Design review of the part shown in the three views and the two pictorial views. Dimensions are in mm from the part's minimum x, y and z. A direction names the side the tool comes from. Coordinates: 2 decimals unless noted, no trailing zeros. Loops run counter-clockwise (first coordinate to the right, second up) from the corner with the lowest first, then second, coordinate; pieces in that order, holes last. Notation, with made-up numbers: (61, -27.75) -> (83, -27.75) arc R28 ccw to (83, 10.25) -> close; hole circle Ø6 at (79, 53). An arc over 180 degrees is marked (long way). One line per item, written item: value.
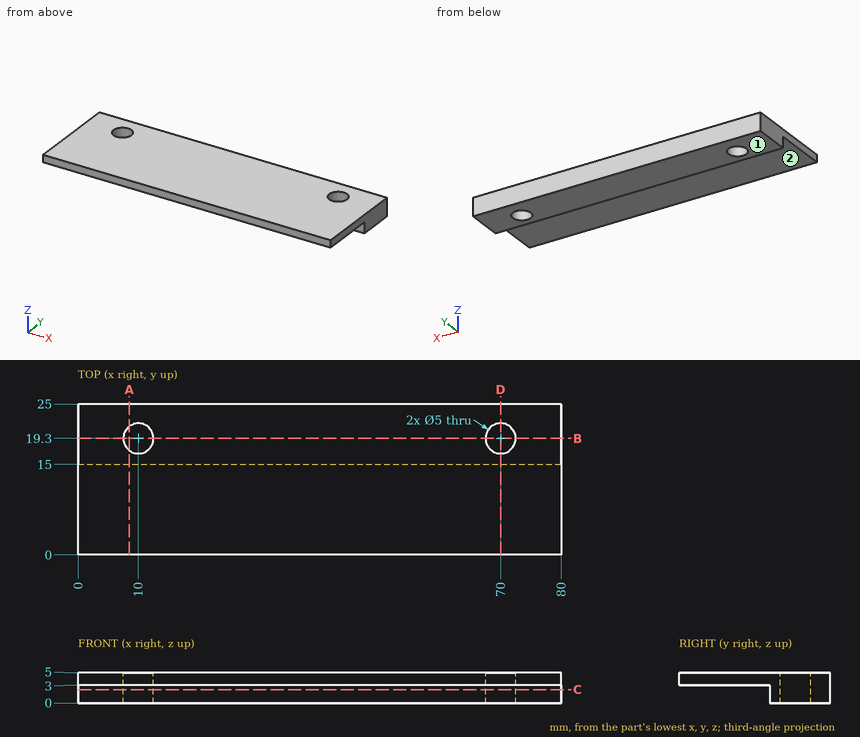
1. To check wall thickness, follow probe 1 along X at (y, z) = (19.3, 1.5); probe 2 along Y at (x, z) = (70, 3.85); probe 3 along Y at (x, z) = (10, 2.6). State the ranges of each line that lie inside material, in increasing order. Write a range as from..to.
Return value:
probe 1: x = 0..7.5, 12.5..67.5, 72.5..80
probe 2: y = 0..16.8, 21.8..25
probe 3: y = 15..16.8, 21.8..25
2. Insertion check: pin 1 Ø7.5 at (x, y) = (38, 5) entering from -Z; pin 2 Ø4 at (x, y) = (10, 19.3) entering from +Z (3 decimals); pin 3 Ø0.9 at (x, z) = (46, 1) entering from -Y. Each pin has a flat end and moves straight along its axis. Give the tip position at first contact, or say it passes through.
Return value:
pin 1: stops at z = 3
pin 2: passes through
pin 3: stops at y = 15
3. Take a section at C-C, the plane z = 2.25. Give the boundary of the cut face in (x, y), and give its area (3 significant figures).
Return value:
outline: (0, 15) -> (80, 15) -> (80, 25) -> (0, 25) -> close; hole circle Ø5 at (10, 19.3); hole circle Ø5 at (70, 19.3)
area: 761 mm2
4. For the marked faces 1 and 2, list the 3-axis set-ups (+Z, -Z, +X, -X, +Y, -Y) from which the entire face can be reached by the end or side of a thin tool; tool diameter is ignored.
Return value:
face 1: -Z, +X, -X, +Y, -Y
face 2: -Z, +X, -X, -Y
5. Take a section at D-D, the plane x = 70. Give the boundary of the cut face in (y, z).
Return value:
outline: (0, 3) -> (15, 3) -> (15, 0) -> (16.8, 0) -> (16.8, 5) -> (0, 5) -> close; (21.8, 0) -> (25, 0) -> (25, 5) -> (21.8, 5) -> close
6. Take a section at B-B, the plane y = 19.3. Give the boundary of the cut face in (x, z).
Return value:
outline: (0, 0) -> (7.5, 0) -> (7.5, 5) -> (0, 5) -> close; (12.5, 0) -> (67.5, 0) -> (67.5, 5) -> (12.5, 5) -> close; (72.5, 0) -> (80, 0) -> (80, 5) -> (72.5, 5) -> close
7. Take a section at A-A, the plane x = 8.5. Give the boundary of the cut face in (y, z), and give its area (3 significant figures).
Return value:
outline: (0, 3) -> (15, 3) -> (15, 0) -> (17.3, 0) -> (17.3, 5) -> (0, 5) -> close; (21.3, 0) -> (25, 0) -> (25, 5) -> (21.3, 5) -> close
area: 60.0 mm2
